from build123d import *

# Parameters (mm, degrees)
SKETCH1_R               = 22
SKETCH1_R_2             = 18
BOSS_EXTRUDE1_DEPTH     = 121
CUT_EXTRUDE2_DEPTH      = 121
CUT_EXTRUDE2_DEPTH_BACK = 121
CUT_EXTRUDE3_DEPTH      = 121
CUT_EXTRUDE3_DEPTH_BACK = 121


with BuildPart() as part:
    # Sketch1 → Boss-Extrude1 (new body)
    with BuildSketch(Plane.XY):
        with BuildLine():
            Line((161.762365998, 18), (-162.025328377, 24.163798034))
            ThreePointArc((-162.025328377, 24.163798034), (-217.498436483, 0.321231462), (-162.5, -24.596747752))
            Line((-162.5, -24.596747752), (161.762365998, -18))
            ThreePointArc((161.762365998, -18), (213.5, 0), (161.762365998, 18))
        make_face()
        with Locations((-184.5, 0)):
            Circle(SKETCH1_R, mode=Mode.SUBTRACT)
        with Locations((184.5, 0)):
            Circle(SKETCH1_R_2, mode=Mode.SUBTRACT)
    extrude(amount=BOSS_EXTRUDE1_DEPTH)

    # Sketch3 → Cut-Extrude2 (cut, two sides: drawn at the far end of the back side and taken through both)
    with BuildSketch(Plane(origin=(1.081289807, 24.960664454, 0), x_dir=(0.9990630180709081, -0.043279162688854546, 0), z_dir=(0.043279162688854546, 0.9990630180709081, 0)).offset(-CUT_EXTRUDE2_DEPTH_BACK)):
        Polygon((-185.755339203, 0), (160.831772656, -7.5), (275.239090967, -7.5), (275.239090967, 54.458825012), (-286.583387746, 54.458825012), (-286.583387746, 0), align=None)
        Polygon((275.239090967, -113.5), (160.831772656, -113.5), (-185.755339203, -121), (-286.583387746, -121), (-286.583387746, -184.896957676), (275.239090967, -184.896957676), align=None)
    extrude(amount=CUT_EXTRUDE2_DEPTH + CUT_EXTRUDE2_DEPTH_BACK, mode=Mode.SUBTRACT)

    # Sketch4 → Cut-Extrude3 (cut, two sides: drawn at the far end of the back side and taken through both)
    with BuildSketch(Plane(origin=(1.081289807, 24.960664454, 0), x_dir=(0.9990630180709081, -0.043279162688854546, 0), z_dir=(0.043279162688854546, 0.9990630180709081, 0)).offset(-CUT_EXTRUDE3_DEPTH_BACK)):
        Polygon((-128.327126834, -60.5), (132.672873166, -60.5), (132.672873166, -42.899081104), (-128.327126834, -37.251150373), align=None)
        Polygon((132.672873166, -60.5), (132.672873166, -78.100918896), (-128.327126834, -83.748849627), (-128.327126834, -60.5), align=None)
    extrude(amount=CUT_EXTRUDE3_DEPTH + CUT_EXTRUDE3_DEPTH_BACK, mode=Mode.SUBTRACT)


solid = part.part
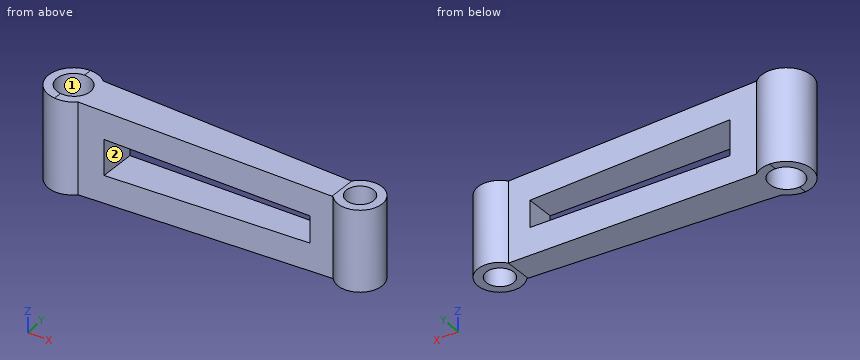
Can you work these out from the model? Positions are in its coordinate system, mm. Face numbers are marked on the shaded views. A direction names the side the tool comes from. Coordinates: 2 decimals unless noted, no trailing zeros. Loops run counter-clockwise (first coordinate to the right, second up) from the corner with the lowest first, then second, coordinate; pieces in that order, holes last. Notation, with made-up numbers: M 15.5,-4 L 36.5,-4 A22 cw 36.5,22 Z; hole C -3.5,-27 d4. An arc over 180 degrees is marked long. Return JSON: item names as keys, results as strings. Group by question number.
Item 1: Imagine slicing it at C-C (x = -60). Please give me the cut outline in (y, z).
Item 2: Imagine slicing it at A-A (x = 184.5). Please give me the cut outline in (y, z), and give its area (3 significant figures).
Item 3: Imagine slicing it at B-B (y = 0). Please give me the cut outline in (x, z).
Item 4: I'm going to push flat-ended pins straight in: pin 1 Ø1.5 at (x, z) = (-22, 13) entering from -Y; pin 2 Ø10 at (y, z) = (1.5, 58) entering from -X; pin 3 Ø10 at (x, y) = (47, -1.5) entering from +Z; pin 4 Ø16 at (x, y) = (175, -1.5) entering from +Z. Where does each tip first touch, or does it pass through?
Item 5: On a 3-axis mill with a long thin cutter (end or side, diameter ignored), from which of +Z, -Z, +X, -X, +Y, -Y can I reach the whole of each face in a straight line? I mean the marked faces 1 and 2. Say none if no direction works.
Item 6: If I drill on L1, parallel to X at y = 15, z = 29; L2, parallel to X at y = -14.5, z = 101; L3, parallel to X at y = -0.5, z = 47, over which ranges is the centre line in solid material (lowest first)? Write a range as from..to.
Verdict:
{
 "1": {"outline": "M -22.51,2.74 L 22.22,2.7 L 22.22,38.71 L -22.51,38.75 Z; M -22.51,82.25 L 22.22,82.29 L 22.22,118.3 L -22.51,118.26 Z"},
 "2": {"outline": "M -29,7.5 L -18,7.5 L -18,113.5 L -29,113.5 Z; M 18,7.5 L 29,7.5 L 29,113.5 L 18,113.5 Z", "area": "2,330 mm^2"},
 "3": {"outline": "M -217.5,0 L -206.5,0 L -206.5,121 L -217.5,121 Z; M -162.5,0.51 L 160.98,7.5 L 166.5,7.5 L 166.5,113.5 L 160.98,113.5 L -162.5,120.49 Z; M 202.5,7.5 L 213.5,7.5 L 213.5,113.5 L 202.5,113.5 Z; hole M -128.45,37.25 L 132.8,42.9 L 132.8,78.1 L -128.45,83.75 Z"},
 "4": {"pin 1": "stops at y = -21.75", "pin 2": "stops at x = -217.5", "pin 3": "stops at z = 116.07", "pin 4": "passes through"},
 "5": {"face 1": "+Z, -Z", "face 2": "-Y"},
 "6": {"L1": "x = -213.89..-200.59, -168.41..174.55, 194.45..209.32", "L2": "x = -214.14..-201.05, -167.95..173.83, 195.17..209.61", "L3": "x = -217.5..-206.49, -162.51..-128.47, 132.78..166.51, 202.49..213.5"}
}
